Autodesk Inventor part; units mm, degrees
ref_plane "YZ Plane" through (0, 0, 0) normal (1, 0, 0) x (0, 1, 0)
ref_plane "XZ Plane" through (0, 0, 0) normal (0, 1, 0) x (-1, 0, 0)
ref_plane "XY Plane" through (0, 0, 0) normal (0, 0, 1) x (1, 0, 0)
sketch "Sketch1" plane through (0, 0, 0) normal (0, 1, 0) x (-1, 0, 0)
  circle A0 centre (0, 0) radius 11
  dimension "d0" = 22
extrude "Extrusion1" add sketch "Sketch1" along normal blind 3.9
sketch "Sketch2" plane through (0, 3.9, 0) normal (0, 1, 0) x (1, 0, 0)
  circle A0 centre (0, 0) radius 9.2
  dimension "d3" = 18.4
extrude "Extrusion2" add sketch "Sketch2" along normal blind 6.55
sketch "Sketch3" plane through (0, 0, 0) normal (0, 0, 1) x (1, 0, 0)
  line L0 (18.8479, 6.1) -> (-23.7231, 6.1)
  line L1 (11, 0) -> (-11, 0)
  line L2 (20.75, 6.1) -> (-20.75, 6.1)
  line L3 (-20.75, 6.1) -> (-20.75, 9.3)
  line L4 (-20.75, 9.3) -> (20.75, 9.3)
  line L5 (20.75, 9.3) -> (20.75, 6.1)
  line L6 (9.2, 10.45) -> (-9.2, 10.45) construction
  line L7 (0, 10.45) -> (0, -1.5119) construction
  point P0 (0, 0)
  point P1 (0, 9.3)
  dimension "d6" = 6.1
  dimension "d7" = 41.5
  dimension "d8" = 3.2
revolve "Revolution1" add sketch "Sketch3" angle 360 about axis through (18.8479, 6.1, 0) along (1, 0, 0)
chamfer "Chamfer1" distance 0.5 angle 45 2 edges at (-20.75, 2.9, 0) (20.75, 2.9, 0)
fillet "Fillet1" radius 0.5 4 edges at (9.8267, 3.9, 2.3238) (9.8267, 3.9, -2.3238) (-9.8267, 3.9, 2.3238) (-9.8267, 3.9, -2.3238)
chamfer "Chamfer2" distance 0.2 angle 45 1 edges at (11, 0, 0)
properties part number "EChem _S200 Cap Top"
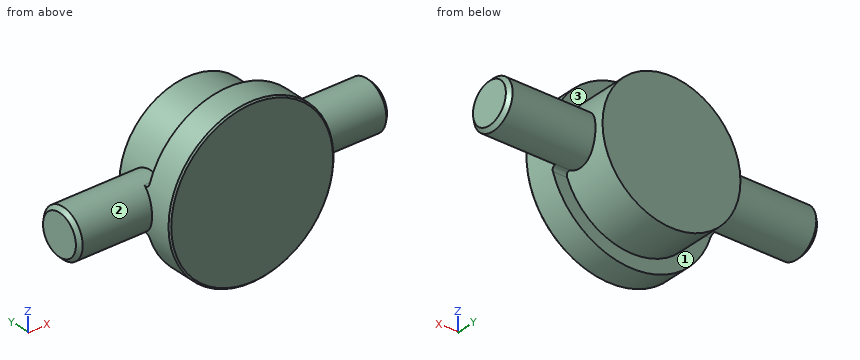
Geometry check sheet. Reference: the model listing, model coordinates, mm. Face numbers are marked on the shaded views. A direction names the side the tool comes from. Coordinates: 2 decimals unless noted, no trailing zeros. Order: outer loops, then holes, each group sorted by start corner. A loop starts at its lowest first (then second) coordinate and runs counter-clockwise, first axis right, second up. Notation, with made-up numbers: M 16,-27 L 74,-27 A17 cw 74,4 Z; hole C -15,-12.5 d1. An arc over 180 degrees is marked long. Answer as a JSON object with one key per item and string values.
Q1. Tool access check on the marked faces 1, 2 and 3. Record the directions out of +Z, -Z, +X, -X, +Y, -Y that give a thin tool (end or side, any length) a straight path to the whole face; none if there is none.
Results are:
{"face 1": "-Z, +Y", "face 2": "-X", "face 3": "+Z, +Y"}
Q2. Cross-section at C-C on x = -13. Record the cut outline in (y, z).
Results are:
{"outline": "C 6.1,0 d6.4"}
Q3. Cross-section at D-D on y = 2.5. Record the cut outline in (x, z).
Results are:
{"outline": "C 0,0 d22"}
Q4. Scan lines: line 1 (Y direction, x = -3, z = -9.5); line 2 (Z direction, x = 13.5, y = 7.5); line 3 (X direction, y = 3.5, z = 1.5). Record each from-to range of solid material in increasing order.
Results are:
{"line 1": "y = 0 to 3.9", "line 2": "z = -2.88 to 2.88", "line 3": "x = -20.45 to 20.45"}
Q5. Depth check by flat-ended pin: pin 1 Ø5 at (x, y) = (0, 6.5) entering from -Z; pin 2 Ø3 at (x, y) = (6, 4.5) entering from -Z; pin 3 Ø2 at (y, z) = (9, 6.5) entering from -X. Enter the tip coordinate at first touch or a pass-through.
Results are:
{"pin 1": "stops at z = -9.2", "pin 2": "stops at z = -9.98", "pin 3": "stops at x = -7.37"}
Q6. Cross-section at A-A on z = 0. Record the cut outline in (x, y).
Results are:
{"outline": "M -20.75,3.4 L -20.25,2.9 L -11,2.9 L -11,0.2 L -10.8,0 L 10.8,0 L 11,0.2 L 11,2.9 L 20.25,2.9 L 20.75,3.4 L 20.75,8.8 L 20.25,9.3 L 9.2,9.3 L 9.2,10.45 L -9.2,10.45 L -9.2,9.3 L -20.25,9.3 L -20.75,8.8 Z"}
Q7. Cross-section at B-B on y = 6.1. Record the cut outline in (x, z), and give its area (3 significant figures).
Results are:
{"outline": "M -20.75,-2.7 L -20.25,-3.2 L -8.63,-3.2 A9.2 ccw 8.63,-3.2 L 20.25,-3.2 L 20.75,-2.7 L 20.75,2.7 L 20.25,3.2 L 8.63,3.2 A9.2 ccw -8.63,3.2 L -20.25,3.2 L -20.75,2.7 Z", "area": "416 mm²"}
